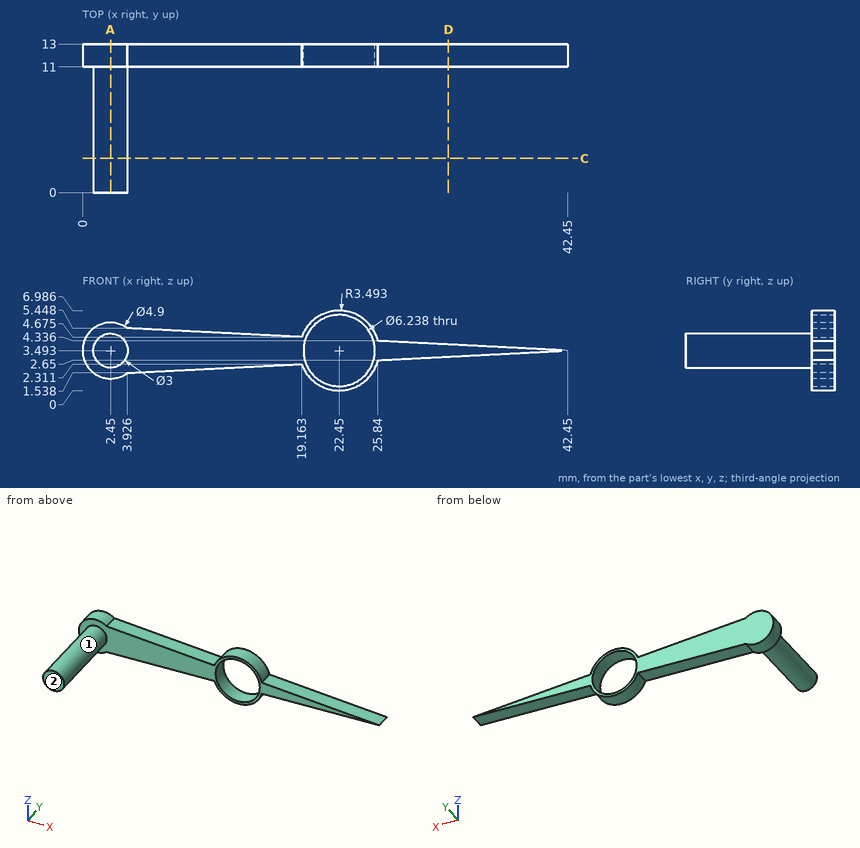
Design review of the part shown in the three views and the two pictorial views. Dimensions are in mm from the part's minimum x, y and z. A direction names the side the tool comes from. Give positions to 0.01 mm unless a question says otherwise; leave off trailing zeros. Write each loop counter-clockwise with the first axis right and the second up, starting at its lowest first coordinate (ties: lowest second). Pieces come first, ordered by that corner, then holes. Notation, with made-up numbers: M 71.25,0.25 L 103.25,0.25 A23 ccw 103.25,30.25 Z; hole C 74.25,-24 d4. An arc over 180 degrees is marked long. Return JSON: item names as keys, results as strings. Group by question number.
Item 1: Clearance check with flat-ended pins moving along their axes: pin 1 Ø1 at (y, z) = (11, 6) entering from +X; pin 2 Ø3.5 at (x, z) = (22.45, 3.49) entering from -Y; pin 3 Ø3 at (y, z) = (2, 3.5) entering from -X; pin 4 Ø2 at (x, z) = (25, 4) entering from -Y. State where each tip first meets the part, or that it passes through.
Item 2: Take a section at A-A (x = 2.45). Give the boundary of the cut face in (y, z).
Item 3: Wall thickness on line 1 along Z through (x, y) = (22.45, 12.15) (1 decimal); line 2 along Y through (x, z) = (7, 1.75); line 3 along Z through (x, y) = (13, 11.75): over which ranges is each line inside the solid? List them lowest first.
Item 4: Tool access review of the marked faces 1 and 2: name each direction out of +Z, -Z, +X, -X, +Y, -Y from which nothing blocks a thin tool from reaching the whole face with its end or side.
Item 5: Take a section at D-D (x = 32). Give the boundary of the cut face in (y, z).
Item 6: Take a section at C-C (y = 3). Give the boundary of the cut face in (x, z).
Return value:
{
 "1": {"pin 1": "stops at x = 25.31", "pin 2": "passes through", "pin 3": "stops at x = 0.95", "pin 4": "stops at y = 11"},
 "2": {"outline": "M 0,1.99 L 11,1.99 L 11,1.04 L 13,1.04 L 13,5.94 L 11,5.94 L 11,4.99 L 0,4.99 Z"},
 "3": {"line 1": "z = 0 to 0.4, 6.6 to 7", "line 2": "y = 11 to 13", "line 3": "z = 2 to 4.99"},
 "4": {"face 1": "-Y", "face 2": "+Z, -Z, +X, -X, -Y"},
 "5": {"outline": "M 11,2.96 L 13,2.96 L 13,4.02 L 11,4.02 Z"},
 "6": {"outline": "C 2.45,3.49 d3"}
}
